Here's the drawing with two shaded views (mm, measured from the low corner). I have some questions. A direction names the side the tool comes from. Give positions to 0.01 mm unless a question says otherwise; leave off trailing zeros. Order: outer loops, then holes, each group sorted by start corner. A loop starts at its lowest first (then second) coordinate and runs counter-clockwise, first axis right, second up. Notation, with made-up numbers: M -5,-19.75 L 50,-19.75 A24 ccw 50,1.25 Z; hole C -40,3 d11. An arc over 180 degrees is marked long. Use a Markdown table: item, result. Add a question column.
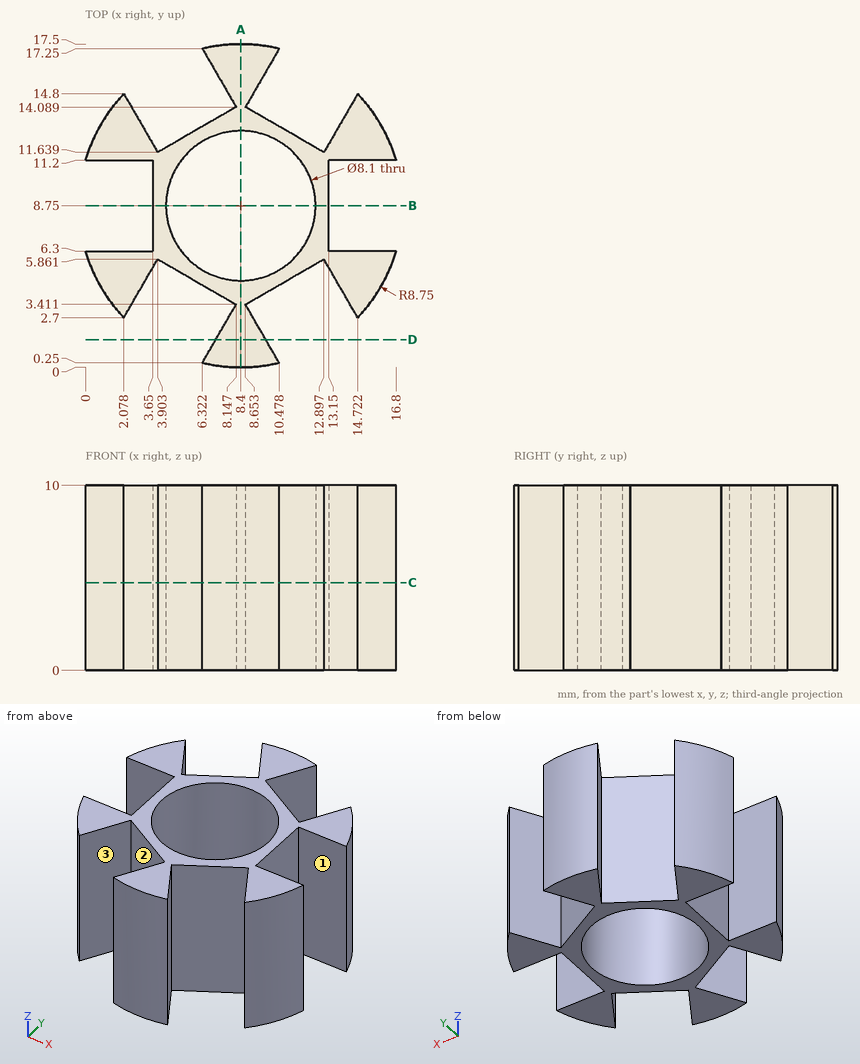
1. If we section it at C-C, the plane z = 4.75: List the corners of the cut face in (x, y) for me.
2. If we section it at B-B, the plane y = 8.75: List the corners of the cut face in (x, z) for me.
3. Will these pins go through, and if not, where does the flat tip stop? pin 1 (1.8 mm diameter, centred on x = 15, z = 4.5, fed in from -Y); pin 2 (3 mm diameter, centred on x = 16, z = 4, fed in from +Y); pin 3 (1.5 mm diameter, centred on y = 15.5, z = 1, fed in from -X); pin 4 (2.5 mm diameter, centred on y = 10, z = 4.5, fed in from -X).
4. I need wall thicknesses on L1, parallel to X at y = 11.75, z = 4.5 (1 decimal); L2, parallel to Y at x = 7.5, z = 2.25 (1 decimal); L3, parallel to Y at x = 9, z = 8.75 (1 decimal). Which ranges of each line are inside material? Lowest first, please. Write a range as [from, to].
5. On a 3-axis mill with a long thin cutter (end or side, diameter ignored), from which of +Z, -Z, +X, -X, +Y, -Y can I reach the whole of each face in a straight line? I mean the marked faces 1, 2 and 3. Say none if no direction works.
6. If we section it at D-D, the plane y = 1.5: List the corners of the cut face in (x, z) for me.
7. If we section it at A-A, the plane x = 8.4: List the corners of the cut face in (y, z) for me.
Geometry results:
| question | item | result |
|---|---|---|
| 1 | outline | M 0,6.3 A8.75 ccw 2.08,2.7 L 3.9,5.86 L 8.15,3.41 L 6.32,0.25 A8.75 ccw 10.48,0.25 L 8.65,3.41 L 12.9,5.86 L 14.72,2.7 A8.75 ccw 16.8,6.3 L 13.15,6.3 L 13.15,11.2 L 16.8,11.2 A8.75 ccw 14.72,14.8 L 12.9,11.64 L 8.65,14.09 L 10.48,17.25 A8.75 ccw 6.32,17.25 L 8.15,14.09 L 3.9,11.64 L 2.08,14.8 A8.75 ccw 0,11.2 L 3.65,11.2 L 3.65,6.3 Z; hole C 8.4,8.75 d8.1 |
| 2 | outline | M 3.65,0 L 4.35,0 L 4.35,10 L 3.65,10 Z; M 12.45,0 L 13.15,0 L 13.15,10 L 12.45,10 Z |
| 3 | pin 1 | stops at y = 2.7 |
| 3 | pin 2 | stops at y = 14.8 |
| 3 | pin 3 | stops at x = 2.03 |
| 3 | pin 4 | stops at x = 0 |
| 4 | L1 | x = [0.2, 3.8], [4.1, 5.7], [11.1, 12.7], [13, 16.6] |
| 4 | L2 | y = [0, 2.3], [3.8, 4.8], [12.7, 13.7], [15.2, 17.5] |
| 4 | L3 | y = [0, 2.8], [3.6, 4.7], [12.8, 13.9], [14.7, 17.5] |
| 5 | face 1 | +Z, -Z, +X |
| 5 | face 2 | +Z, -Z |
| 5 | face 3 | +Z, -Z, -Y |
| 6 | outline | M 7.04,0 L 9.76,0 L 9.76,10 L 7.04,10 Z |
| 7 | outline | M 0,0 L 4.7,0 L 4.7,10 L 0,10 Z; M 12.8,0 L 17.5,0 L 17.5,10 L 12.8,10 Z |
